Check sheet for the modelled part. Datum: model origin and axes. Units: mm. Face numbers are marked on the shaded views. A direction names the side the tool comes from. Coordinates: 2 decimals unless noted, no trailing zeros. Order: outer loops, then holes, each group sorted by start corner. A loop starts at its lowest first (then second) coordinate and runs counter-clockwise, first axis right, second up. Notation, with made-up numbers: M -39,45 L -35,45 A6 ccw -35,53 Z; hole C 66,-9 d11. An arc over 180 degrees is marked long. Answer in a Markdown table with one row per item. Add a question column.
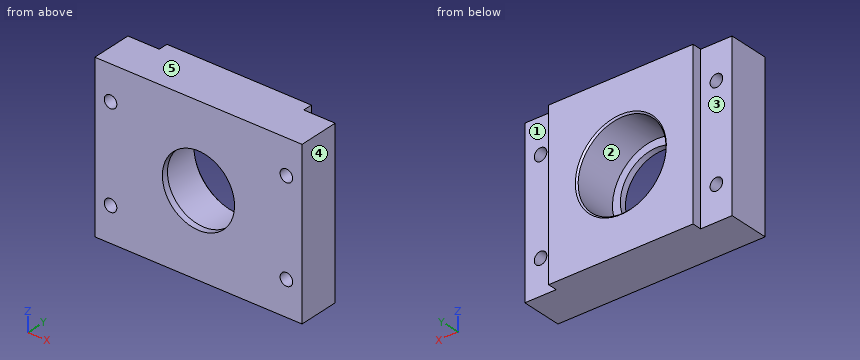
from build123d import *

# Parameters (mm, degrees)
SKETCH_1_W          = 50
SKETCH_1_H          = 52
SKETCH_1_R          = 14
EXTRUDE_1_DEPTH     = 16
SKETCH_2_R          = 14
SKETCH_2_R_2        = 11.5
EXTRUDE_2_DEPTH     = 2
SKETCH_3_W          = 8
SKETCH_3_H          = 13
EXTRUDE_3_DEPTH     = 52
SKETCH_4_R          = 2
CUT_EXTRUDE_1_DEPTH = 44.977266855
CHAMFER_1_SIZE      = 0.5
SKETCH_5_W          = 2
SKETCH_5_H          = 3
CUT_EXTRUDE_2_DEPTH = 64.63175308


with BuildPart() as part:
    # 草图1 → 凸台-拉伸1 (new body)
    with BuildSketch(Plane(origin=(0, 0, 0), x_dir=(1, 0, 0), z_dir=(0, 1, 0))):
        Rectangle(SKETCH_1_W, SKETCH_1_H)
        with Locations(Location((0, 0, 0), (0, 0, 270))):
            Circle(SKETCH_1_R, mode=Mode.SUBTRACT)
    extrude(amount=EXTRUDE_1_DEPTH)

    # 草图2 → 凸台-拉伸2 (add)
    with BuildSketch(Plane.XZ):
        with Locations(Location((0, 0, 0), (0, 0, 270))):
            Circle(SKETCH_2_R)
        with Locations(Location((0, 0, 0), (0, 0, 270))):
            Circle(SKETCH_2_R_2, mode=Mode.SUBTRACT)
    extrude(amount=-EXTRUDE_2_DEPTH)

    # 草图3 → 凸台-拉伸3 (add)
    with BuildSketch(Plane(origin=(0, 0, -26), x_dir=(-1, 0, 0), z_dir=(0, 0, -1))):
        with Locations((-29, 6.5)):
            Rectangle(SKETCH_3_W, SKETCH_3_H)
        with Locations((29, 6.5)):
            Rectangle(SKETCH_3_W, SKETCH_3_H)
    extrude(amount=-EXTRUDE_3_DEPTH)

    # 草图4 → 切除-拉伸1 (cut, through all)
    with BuildSketch(Plane(origin=(0, 13, 0), x_dir=(1, 0, 0), z_dir=(0, 1, 0))):
        with Locations(Location((-28, 15, 0), (0, 0, 180))):
            Circle(SKETCH_4_R)
        with Locations(Location((-28, -15, 0), (0, 0, 180))):
            Circle(SKETCH_4_R)
        with Locations(Location((28, 15, 0), (0, 0, 180))):
            Circle(SKETCH_4_R)
        with Locations(Location((28, -15, 0), (0, 0, 180))):
            Circle(SKETCH_4_R)
    extrude(amount=-CUT_EXTRUDE_1_DEPTH, mode=Mode.SUBTRACT)

    # 倒角1
    chamfer_1_edges = [part.edges().sort_by_distance(p)[0] for p in [
        (0, 16, -14),
    ]]
    chamfer(chamfer_1_edges, length=CHAMFER_1_SIZE)

    # 草图5 → 切除-拉伸2 (cut, through all)
    with BuildSketch(Plane.XY.offset(26)):
        with Locations((-24, 14.5)):
            Rectangle(SKETCH_5_W, SKETCH_5_H)
        with Locations((24, 14.5)):
            Rectangle(SKETCH_5_W, SKETCH_5_H)
    extrude(amount=-CUT_EXTRUDE_2_DEPTH, mode=Mode.SUBTRACT)


solid = part.part
1. Section check B-B on z = 0. Enter the section's corners in (x, y), then the cut area to 3 significant figures.
2. Section check D-D on y = 14.25. Enter the section's corners in (x, z).
3. Section check A-A on x = 0. Enter the section's corners in (y, z), then the cut area to 3 significant figures.
4. Go/stop test with flat-tipped pins: pin 1 Ø0.9 at (y, z) = (14.5, -1) entering from -X; pin 2 Ø0.9 at (y, z) = (14.5, -11.5) entering from +X; pin 3 Ø8 at (x, z) = (-28, -9.5) entering from +Y. Record where each tip stops, or that it passes through.
5. Scan lines: line 1 (Z direction, x = 28, y = 8.5); line 2 (Z direction, x = 11, y = 10.25); line 3 (X direction, y = 5.5, z = -4). Record each from-to range of solid material in increasing order.
6. Section check C-C on x = -28. Enter the section's corners in (y, z).
7. Set-up check for the marked faces 1, 2, 3, 4 and 5: record each of +Z, -Z, +X, -X, +Y, -Y from which the full face is reachable in a straight line by a thin tool's end or side.
Result sheet:
| question | item | result |
|---|---|---|
| 1 | outline | M -33,0 L -11.5,0 L -11.5,2 L -14,2 L -14,15.5 L -14.5,16 L -23,16 L -23,13 L -33,13 Z; M 11.5,0 L 33,0 L 33,13 L 23,13 L 23,16 L 14.5,16 L 14,15.5 L 14,2 L 11.5,2 Z |
| 1 | area | 558 mm^2 |
| 2 | outline | M -23,-26 L 23,-26 L 23,26 L -23,26 Z; hole C 0,0 d28 |
| 3 | outline | M 0,-26 L 16,-26 L 16,-14.5 L 15.5,-14 L 2,-14 L 2,-11.5 L 0,-11.5 Z; M 0,11.5 L 2,11.5 L 2,14 L 15.5,14 L 16,14.5 L 16,26 L 0,26 Z |
| 3 | area | 394 mm^2 |
| 4 | pin 1 | x = -23 |
| 4 | pin 2 | x = 23 |
| 4 | pin 3 | y = 13 |
| 5 | line 1 | -26 to -17, -13 to 13, 17 to 26 |
| 5 | line 2 | -26 to -8.66, 8.66 to 26 |
| 5 | line 3 | -33 to -13.42, 13.42 to 33 |
| 6 | outline | M 0,-26 L 13,-26 L 13,-17 L 0,-17 Z; M 0,-13 L 13,-13 L 13,13 L 0,13 Z; M 0,17 L 13,17 L 13,26 L 0,26 Z |
| 7 | face 1 | +Z, -Z, +X, +Y |
| 7 | face 2 | +Y |
| 7 | face 3 | +Z, -Z, -X, +Y |
| 7 | face 4 | +Z, -Z, +X, +Y, -Y |
| 7 | face 5 | +Z, +X, -X, +Y, -Y |
